Part print with two shaded views. Sizes in mm from the minimum x, y, z corner. Round coordinates to 2 decimals unless told otherwise and drop trailing zeros. Write each loop counter-clockwise with the first axis right and the second up, starting at its lowest first coordinate (ties: lowest second). Pieces come first, ordered by that corner, then holes. Notation, with made-up numbers: (9, 11.25) -> (46, 11.25) arc R28 ccw to (46, 46.25) -> close; hole circle Ø4 at (49.25, 73.25). An arc over 180 degrees is marked (long way). Return JSON: item names as keys, results as strings. Group by question number.
(1) Saw through at C-C (z = 18.5). List the corners of the cut face in (x, y), plus the area to 3 significant figures.
(2) Drill centre lines: L1, parallel to Z at x = 20, y = 17.75; L2, parallel to Y at x = 6, z = 17.25; L3, parallel to X at y = 8.75, z = 12.5. Where is each one in solid material? Low to high. Write a range as from..to.
(3) Saw through at A-A (y = 12). List the corners of the cut face in (x, z).
(4) Saw through at B-B (x = 6). List the corners of the cut face in (y, z).
(5) Mould opens along Y. For the marked faces 1, 2 and 3 say: +Y half, -Y half, draft (parallel to the pull), parting line (faces both ways), or undercut.
(6) Drop flat-ended pins along their axis: pin 1 Ø6 at (y, z) = (5.5, 10.5) entering from -X; pin 2 Ø9 at (x, z) = (20, 12.5) entering from +Y. Give the stop position or say it passes through.
(7) Saw through at D-D (z = 2). List the corners of the cut face in (x, y), plus the area to 3 significant figures.
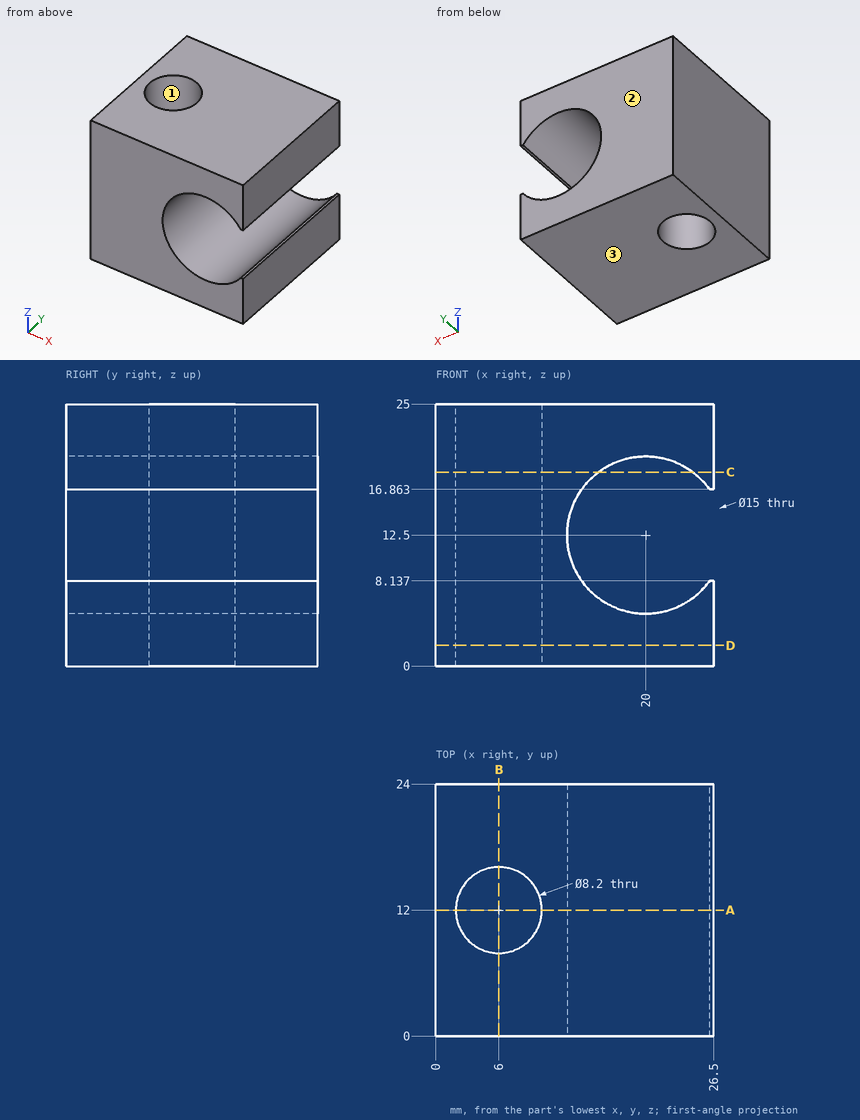
Computed values:
{
 "1": {"outline": "(0, 0) -> (15.5, 0) -> (15.5, 24) -> (0, 24) -> close; (24.5, 0) -> (26.5, 0) -> (26.5, 24) -> (24.5, 24) -> close; hole circle Ø8.2 at (6, 12)", "area": "367 mm2"},
 "2": {"L1": "0..5, 20..25", "L2": "0..7.9, 16.1..24", "L3": "0..3.5, 8.5..12.5"},
 "3": {"outline": "(0, 0) -> (1.9, 0) -> (1.9, 25) -> (0, 25) -> close; (10.1, 0) -> (26.5, 0) -> (26.5, 8.14) -> (26.1, 8.14) arc R7.5 cw (long way) to (26.1, 16.86) -> (26.5, 16.86) -> (26.5, 25) -> (10.1, 25) -> close"},
 "4": {"outline": "(0, 0) -> (7.9, 0) -> (7.9, 25) -> (0, 25) -> close; (16.1, 0) -> (24, 0) -> (24, 25) -> (16.1, 25) -> close"},
 "5": {"face 1": "undercut", "face 2": "+Y half", "face 3": "draft"},
 "6": {"pin 1": "x = 0", "pin 2": "through"},
 "7": {"outline": "(0, 0) -> (26.5, 0) -> (26.5, 24) -> (0, 24) -> close; hole circle Ø8.2 at (6, 12)", "area": "583 mm2"}
}
